Geometry: final body of the model. Coordinates: model frame, mm. Round coordinates to 2 decimals unless told otherwise and drop trailing zeros. Write each loop counter-clockwise with the first axis right and the second up, starting at its lowest first coordinate (ties: lowest second). Pieces come first, ordered by that corner, then holes.
from build123d import *

# Parameters (mm, degrees)
SKETCH1_W           = 78
SKETCH1_H           = 3.498668771
BOSS_EXTRUDE1_DEPTH = 140
FILLET1_R           = 8
CUT_EXTRUDE1_DEPTH  = 10


with BuildPart() as part:
    # Sketch1 → Boss-Extrude1 (new body)
    with BuildSketch(Plane(origin=(468.829800242, 0, 0), x_dir=(0, 0, -1), z_dir=(1, 0, 0))):
        with Locations((-329.624739584, 1.749334386)):
            Rectangle(SKETCH1_W, SKETCH1_H)
    extrude(amount=-BOSS_EXTRUDE1_DEPTH)

    # Fillet1
    fillet1_edges = [part.edges().sort_by_distance(p)[0] for p in [
        (468.829800242, 1.749334385, 290.624739584),
        (328.829800242, 1.749334385, 290.624739584),
        (328.829800242, 1.749334385, 368.624739584),
        (468.829800242, 1.749334385, 368.624739584),
    ]]
    fillet(fillet1_edges, radius=FILLET1_R)

    # Sketch3 → Cut-Extrude1 (cut)
    with BuildSketch(Plane(origin=(0, 3.498668771, 0), x_dir=(1, 0, 0), z_dir=(0, 1, 0))):
        with BuildLine():
            Line((353.079800242, -345.374739584), (444.579800242, -345.374739584))
            ThreePointArc((444.579800242, -345.374739584), (448.829800242, -349.624739584), (444.579800242, -353.874739584))
            Line((444.579800242, -353.874739584), (353.079800242, -353.874739584))
            ThreePointArc((353.079800242, -353.874739584), (348.829800242, -349.624739584), (353.079800242, -345.374739584))
        make_face()
        with BuildLine():
            Line((353.079800242, -305.374739584), (444.579800242, -305.374739584))
            ThreePointArc((444.579800242, -305.374739584), (448.829800242, -309.624739584), (444.579800242, -313.874739584))
            Line((444.579800242, -313.874739584), (353.079800242, -313.874739584))
            ThreePointArc((353.079800242, -313.874739584), (348.829800242, -309.624739584), (353.079800242, -305.374739584))
        make_face()
    extrude(amount=-CUT_EXTRUDE1_DEPTH, mode=Mode.SUBTRACT)


solid = part.part
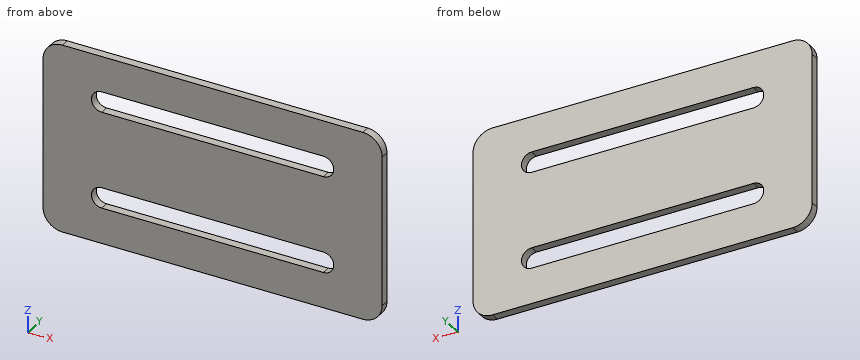
1) Section B-B on y = 0.85. Output: boundary loops of the cut face in (x, z).
2) Line query: probe 1 along Z at (x, y) = (442.5, 0.7); probe 2 along Z at (x, y) = (446.5, 2.85); probe 3 along X at (y, z) = (1.75, 350). Output: solid intervals per line, ascending.
3) Section C-C on z = 349.5. Output: boundary loops of the cut face in (x, y).
4) Section A-A on x = 439. Output: boundary loops of the cut face in (y, z).
Filled in:
1. outline: (328.83, 298.62) arc R8 ccw to (336.83, 290.62) - (460.83, 290.62) arc R8 ccw to (468.83, 298.62) - (468.83, 360.62) arc R8 ccw to (460.83, 368.62) - (336.83, 368.62) arc R8 ccw to (328.83, 360.62) - close; hole (353.08, 305.37) - (444.58, 305.37) arc R4.25 ccw to (444.58, 313.87) - (353.08, 313.87) arc R4.25 ccw to start; hole (353.08, 345.37) - (444.58, 345.37) arc R4.25 ccw to (444.58, 353.87) - (353.08, 353.87) arc R4.25 ccw to start
2. probe 1: z = 290.62 to 305.37, 313.87 to 345.37, 353.87 to 368.62
2. probe 2: z = 290.62 to 305.83, 313.42 to 345.83, 353.42 to 368.62
2. probe 3: x = 328.83 to 348.85, 448.81 to 468.83
3. outline: (328.83, 0) - (348.83, 0) - (348.83, 3.5) - (328.83, 3.5) - close; (448.83, 0) - (468.83, 0) - (468.83, 3.5) - (448.83, 3.5) - close
4. outline: (0, 290.62) - (3.5, 290.62) - (3.5, 305.37) - (0, 305.37) - close; (0, 313.87) - (3.5, 313.87) - (3.5, 345.37) - (0, 345.37) - close; (0, 353.87) - (3.5, 353.87) - (3.5, 368.62) - (0, 368.62) - close
